CAD build for the part. Positions are in the model's coordinates, mm. A direction names the side the tool comes from. Give positions to 0.01 mm unless a question says otherwise; leave off trailing zeros. Write each loop counter-clockwise with the first axis right and the second up, starting at its lowest first coordinate (ties: lowest second). Pieces come first, ordered by that corner, then holes. Notation, with made-up numbers: M 15.25,38.5 L 37.25,38.5 A21 cw 37.25,58.5 Z; hole C 81.25,-10.75 d6. An arc over 180 degrees is marked long. One line per question, with ' | ' between items. Start each with the question number.
1. Cut at B-B, the plane x = 5. Write the cut outline in (y, z).
2. Cut at A-A, the plane z = -37.95. Write the cut outline in (x, y).
3. Cut at D-D, the plane z = -15. Write the cut outline in (x, y).
4. Pull direction Z, two halves, no side cores. Call faces 5 (the face through (6, 0, 22.75)), 6 (the face through (17, 21, -25.25)), 7 (the face through (6, 19.55, -16)): released by +Z, released by -Z, zero draft, split by the parting line, or undercut.
5. Which spindle directions (+Z, -Z, +X, -X, +Y, -Y) get a long thin tool onto all of the face, cutting with end or side? Do faces 1 (the face through (7.2, -18.8, -27.15)), 2 (the face through (10.47, 19, 6)), 3 (the face through (1, 15.35, -13)), 4 (the face through (14, 16.55, 11)). Say none if no direction does.
6. Wall check: L1, parallel to Z at x = 14.47, y = -18; L2, parallel to Y at x = 12.8, z = -24.7; L3, parallel to Z at x = 14.47, y = 18.5. Give the ranges that are in metal, low to high.
7. Cut at C-C, the plane y = 7. Write the cut outline in (x, z).
8. Flat gauge pins, fed straight in: pin 1 (3.5 mm diameter, centred on y = 22.85, z = -37.95, fed in from +X); pin 2 (3 mm diameter, centred on y = 15.5, z = -13.5, fed in from +X); pin 3 (8.5 mm diameter, centred on x = 14.5, y = -9, fed in from -Z); pin 4 (0.8 mm diameter, centred on x = 21.5, z = -23.5, fed in from -Y). Where does each tip first touch, or does it go through?
```python
from build123d import *

# Parameters (mm, degrees)
CROQUIS4_W              = 45.5
CROQUIS4_H              = 45.3
SALIENTE_EXTRUIR3_DEPTH = 21.47
CROQUIS5_W              = 41.141731218
CROQUIS5_H              = 30.7
CORTAR_EXTRUIR2_DEPTH   = 18.77
CROQUIS6_W              = 18.6
CROQUIS6_H              = 24.6
CORTAR_EXTRUIR3_DEPTH   = 18.77
CROQUIS7_R              = 3
CORTAR_EXTRUIR4_DEPTH   = 58.77
CROQUIS8_R              = 6.02
CORTAR_EXTRUIR5_DEPTH   = 58.77
CROQUIS9_W              = 6
CROQUIS9_H              = 16.319841708
CORTAR_EXTRUIR7_DEPTH   = 1.2
CHAFL_N1_SIZE           = 1.2
CROQUIS10_W             = 8
CROQUIS10_H             = 5
CORTAR_EXTRUIR8_DEPTH   = 71.2
CROQUIS11_W             = 6
CROQUIS11_H             = 16.418152186
CORTAR_EXTRUIR9_DEPTH   = 1.2
CHAFL_N2_SIZE           = 1.2
CORTAR_EXTRUIR12_DEPTH  = 11.2
CORTAR_EXTRUIR14_DEPTH  = 7
CROQUIS15_W             = 12.3
CROQUIS15_H             = 4.2
CORTAR_EXTRUIR15_DEPTH  = 9.47
CROQUIS16_W             = 7
CROQUIS16_H             = 5
CORTAR_EXTRUIR17_DEPTH  = 0.3
CROQUIS17_W             = 7
CROQUIS17_H             = 0.8
SALIENTE_EXTRUIR4_DEPTH = 3
CROQUIS18_W             = 21.819351721
CROQUIS18_H             = 12.3
CORTAR_EXTRUIR18_DEPTH  = 53
SALIENTE_EXTRUIR5_START = -2.7
CROQUIS19_W             = 24
CROQUIS19_H             = 41.5
SALIENTE_EXTRUIR5_DEPTH = 6.8
CROQUIS21_W             = 2.5
CROQUIS21_H             = 10.5
SALIENTE_EXTRUIR6_DEPTH = 20.5
CROQUIS22_R             = 1.95
CORTAR_EXTRUIR19_DEPTH  = 20.5
CROQUIS23_W             = 9.795322327
CROQUIS23_H             = 20.802243728
CORTAR_EXTRUIR20_DEPTH  = 20.5
CROQUIS24_R             = 1.1
CORTAR_EXTRUIR22_DEPTH  = 2.5
CROQUIS25_W             = 2.17
CROQUIS25_H             = 12.3
CORTAR_EXTRUIR23_DEPTH  = 13
CROQUIS26_R             = 3
CORTAR_EXTRUIR24_DEPTH  = 2.5
SALIENTE_EXTRUIR7_REACH = 70.642
CROQUIS31_W             = 4.4
CROQUIS31_H             = 7.8
SALIENTE_EXTRUIR8_DEPTH = 8.7
CROQUIS32_R             = 3
CORTAR_EXTRUIR25_DEPTH  = 8.7


# Some blends are built 0.0001 mm under size
with BuildPart() as part:
    # Croquis4 → Saliente-Extruir3 (new body)
    with BuildSketch(Plane(origin=(0, 0, 0), x_dir=(0, 0, -1), z_dir=(1, 0, 0))):
        Rectangle(CROQUIS4_W, CROQUIS4_H)
    extrude(amount=SALIENTE_EXTRUIR3_DEPTH)

    # Croquis5 → Cortar-Extruir2 (cut)
    with BuildSketch(Plane(origin=(21.47, 0, 0), x_dir=(0, 0, -1), z_dir=(1, 0, 0))):
        with Locations((2.520865609, 0)):
            Rectangle(CROQUIS5_W, CROQUIS5_H)
    extrude(amount=-CORTAR_EXTRUIR2_DEPTH, mode=Mode.SUBTRACT)

    # Croquis6 → Cortar-Extruir3 (cut)
    with BuildSketch(Plane(origin=(0, 22.65, 0), x_dir=(1, 0, 0), z_dir=(0, 1, 0))):
        with Locations((21.47, 22.75)):
            Rectangle(CROQUIS6_W, CROQUIS6_H)
    extrude(amount=-CORTAR_EXTRUIR3_DEPTH, mode=Mode.SUBTRACT)

    # Croquis7 → Cortar-Extruir4 (cut)
    with BuildSketch(Plane(origin=(0, 22.65, 0), x_dir=(1, 0, 0), z_dir=(0, 1, 0))):
        with Locations(Location((14.47, -17.25, 0), (0, 0, 270))):
            Circle(CROQUIS7_R)
        with Locations(Location((14.47, 4.95, 0), (0, 0, 270))):
            Circle(CROQUIS7_R)
    extrude(amount=-CORTAR_EXTRUIR4_DEPTH, mode=Mode.SUBTRACT)

    # Croquis8 → Cortar-Extruir5 (cut)
    with BuildSketch(Plane.XY.offset(22.75)):
        with Locations((12.7, 0)):
            Circle(CROQUIS8_R)
    extrude(amount=-CORTAR_EXTRUIR5_DEPTH, mode=Mode.SUBTRACT)

    # Croquis9 → Cortar-Extruir7 (cut)
    with BuildSketch(Plane.XZ.offset(-15.35)):
        with Locations((14.47, 6.060847086)):
            Rectangle(CROQUIS9_W, CROQUIS9_H)
    extrude(amount=-CORTAR_EXTRUIR7_DEPTH, mode=Mode.SUBTRACT)

    # Chaflán1
    # the kernel refuses this chamfer: 1.2 mm, written as the material it takes off along each edge
    with BuildSketch(Plane(origin=(12.317907402, 15.35, -2.099073768), x_dir=(0, -0.027495876610584495, -0.9996219169112968), z_dir=(1, 0, 0)), Plane(origin=(11.47, 15.35, -2.099073768), x_dir=(0, -0.027495876610584533, -0.9996219169112968), z_dir=(1, 0, 0))) as chafl_n1_piece_1:
        Polygon((CHAFL_N1_SIZE * 0.999621916911, CHAFL_N1_SIZE * 0.0274958766106), (-CHAFL_N1_SIZE * 0.0274958766106, CHAFL_N1_SIZE * 0.999621916911), (0, 0), align=None)
    extrude(amount=5.152092598, mode=Mode.SUBTRACT)
    with BuildSketch(Plane(origin=(17.47, 15.35, 14.22076794), x_dir=(0, -0.027495876610585984, 0.9996219169112968), z_dir=(-1, 0, 0))) as chafl_n1_piece_2_section:
        Polygon((CHAFL_N1_SIZE * 0.999621916911, CHAFL_N1_SIZE * 0.0274958766106), (-CHAFL_N1_SIZE * 0.0274958766106, CHAFL_N1_SIZE * 0.999621916911), (0, 0), align=None)
    chafl_n1_piece_2 = extrude(amount=6, mode=Mode.PRIVATE)
    chafl_n1_piece_2 = split(chafl_n1_piece_2, bisect_by=Plane(origin=(14.47, 16.55, 14.617252925), z_dir=(0, -1, 0)), keep=Keep.TOP, mode=Mode.PRIVATE)
    add(chafl_n1_piece_2, mode=Mode.SUBTRACT)

    # Croquis10 → Cortar-Extruir8 (cut)
    with BuildSketch(Plane(origin=(0, 22.65, 0), x_dir=(1, 0, 0), z_dir=(0, 1, 0))):
        with Locations((14.47, -6.15)):
            Rectangle(CROQUIS10_W, CROQUIS10_H)
    extrude(amount=-CORTAR_EXTRUIR8_DEPTH, mode=Mode.SUBTRACT)

    # Croquis11 → Cortar-Extruir9 (cut)
    with BuildSketch(Plane(origin=(0, -15.35, 0), x_dir=(1, 0, 0), z_dir=(0, 1, 0))):
        with Locations((14.47, -6.15)):
            Rectangle(CROQUIS11_W, CROQUIS11_H)
    extrude(amount=-CORTAR_EXTRUIR9_DEPTH, mode=Mode.SUBTRACT)

    # Chaflán2
    chafl_n2_edges = [part.edges().sort_by_distance(p)[0] for p in [
        (12.569201122, -15.35, -2.059076093),
        (16.370798878, -15.35, -2.059076093),
        (12.569201122, -15.35, 14.359076093),
        (16.370798878, -15.35, 14.359076093),
    ]]
    chamfer(chafl_n2_edges, length=CHAFL_N2_SIZE - 0.0001)  # a hair under: the kernel refuses the full size

    # Croquis12 → Cortar-Extruir12 (cut)
    with BuildSketch(Plane(origin=(2.7, 0, 0), x_dir=(0, 0, -1), z_dir=(1, 0, 0))):
        Polygon((8.65, 15.35), (8.65, -15.35), (11.55469898, -15.35), (11.55469898, -14.35), (18.45, -14.35), (18.45, 15.35), align=None)
    extrude(amount=-CORTAR_EXTRUIR12_DEPTH, mode=Mode.SUBTRACT)

    # Croquis14 → Cortar-Extruir14 (cut)
    with BuildSketch(Plane(origin=(2.7, 0, 0), x_dir=(0, 0, -1), z_dir=(1, 0, 0))):
        Polygon((10.15, 15.35), (5.15, 15.35), (10.15, 20.35), align=None)
    extrude(amount=CORTAR_EXTRUIR14_DEPTH, mode=Mode.SUBTRACT)

    # Croquis15 → Cortar-Extruir15 (cut)
    with BuildSketch(Plane(origin=(12.17, 0, 0), x_dir=(0, 0, -1), z_dir=(1, 0, 0))):
        with Locations((16.6, 17.45)):
            Rectangle(CROQUIS15_W, CROQUIS15_H)
    extrude(amount=-CORTAR_EXTRUIR15_DEPTH, mode=Mode.SUBTRACT)

    # Croquis16 → Cortar-Extruir17 (cut)
    with BuildSketch(Plane.XY.offset(-10.15)):
        with Locations((6.2, 17.85)):
            Rectangle(CROQUIS16_W, CROQUIS16_H)
    extrude(amount=-CORTAR_EXTRUIR17_DEPTH, mode=Mode.SUBTRACT)

    # Croquis17 → Saliente-Extruir4 (add)
    with BuildSketch(Plane(origin=(0, 0, -10.45), x_dir=(-1, 0, 0), z_dir=(0, 0, -1))):
        with Locations((-6.2, 19.95)):
            Rectangle(CROQUIS17_W, CROQUIS17_H)
    extrude(amount=-SALIENTE_EXTRUIR4_DEPTH)

    # Croquis18 → Cortar-Extruir18 (cut)
    with BuildSketch(Plane.XZ.offset(-19.55)):
        with Locations((13.609675861, -16.6)):
            Rectangle(CROQUIS18_W, CROQUIS18_H)
    extrude(amount=CORTAR_EXTRUIR18_DEPTH, mode=Mode.SUBTRACT)

    # Croquis19 → Saliente-Extruir5 (add)
    with BuildSketch(Plane(origin=(2.7, 0, 0), x_dir=(0, 0, -1), z_dir=(1, 0, 0)).offset(SALIENTE_EXTRUIR5_START)):
        with Locations((34.75, 5.9)):
            Rectangle(CROQUIS19_W, CROQUIS19_H)
    extrude(amount=SALIENTE_EXTRUIR5_DEPTH)

    # Croquis21 → Saliente-Extruir6 (add)
    with BuildSketch(Plane(origin=(6.8, 0, 0), x_dir=(0, 0, -1), z_dir=(1, 0, 0))):
        with Locations((24, 21.4)):
            Rectangle(CROQUIS21_W, CROQUIS21_H)
        with Locations((24, -9.6)):
            Rectangle(CROQUIS21_W, CROQUIS21_H)
    extrude(amount=SALIENTE_EXTRUIR6_DEPTH)

    # Croquis22 → Cortar-Extruir19 (cut)
    with BuildSketch(Plane(origin=(6.8, 0, 0), x_dir=(0, 0, -1), z_dir=(1, 0, 0))):
        with Locations((37.95, 22.85)):
            Circle(CROQUIS22_R)
        with Locations((37.95, -11.05)):
            Circle(CROQUIS22_R)
    extrude(amount=-CORTAR_EXTRUIR19_DEPTH, mode=Mode.SUBTRACT)

    # Croquis23 → Cortar-Extruir20 (cut)
    with BuildSketch(Plane(origin=(0, 0, -10.45), x_dir=(-1, 0, 0), z_dir=(0, 0, -1))):
        with Locations((-26.367661164, -11.870604275)):
            Rectangle(CROQUIS23_W, CROQUIS23_H)
    extrude(amount=CORTAR_EXTRUIR20_DEPTH, mode=Mode.SUBTRACT)

    # Croquis24 → Cortar-Extruir22 (cut)
    with BuildSketch(Plane(origin=(0, 0, -25.25), x_dir=(-1, 0, 0), z_dir=(0, 0, -1))):
        with Locations((-12.8, -9.25)):
            Circle(CROQUIS24_R)
        with Locations((-12.8, 19.15)):
            Circle(CROQUIS24_R)
    extrude(amount=-CORTAR_EXTRUIR22_DEPTH, mode=Mode.SUBTRACT)

    # Croquis25 → Cortar-Extruir23 (cut)
    with BuildSketch(Plane.XZ.offset(-19.55)):
        with Locations((11.085, -16.6)):
            Rectangle(CROQUIS25_W, CROQUIS25_H)
    extrude(amount=-CORTAR_EXTRUIR23_DEPTH, mode=Mode.SUBTRACT)

    # Croquis26 → Cortar-Extruir24 (cut)
    with BuildSketch(Plane(origin=(0, 0, -25.25), x_dir=(-1, 0, 0), z_dir=(0, 0, -1))):
        with Locations(Location((-22.05, 21.4, 0), (0, 0, 90))):
            Circle(CROQUIS26_R)
    extrude(amount=-CORTAR_EXTRUIR24_DEPTH, mode=Mode.SUBTRACT)

    # Saliente-Extruir7: up to this face of the body (flat: up to its plane)
    saliente_extruir7_end = Plane(part.part.faces().sort_by_distance((9.699863726, -22.65, 4.986693104))[0])
    # Croquis30 → Saliente-Extruir7 (add, up to the picked face)
    with BuildSketch(Plane.XZ.offset(-19.55), mode=Mode.PRIVATE) as saliente_extruir7_sk1:
        Polygon((2.7, -18.45), (6.8, -22.75), (2.7, -22.75), align=None)
    saliente_extruir7_tool1 = split(extrude(saliente_extruir7_sk1.sketch, amount=SALIENTE_EXTRUIR7_REACH, mode=Mode.PRIVATE), bisect_by=saliente_extruir7_end, keep=Keep.BOTH, mode=Mode.PRIVATE)
    add(saliente_extruir7_tool1.solids().sort_by(Axis((4.066667, 19.55, -21.316667), (0, -1, 0)))[0])

    # Croquis31 → Saliente-Extruir8 (add)
    with BuildSketch(Plane.ZY):
        with Locations((-24.95, -18.75)):
            Rectangle(CROQUIS31_W, CROQUIS31_H)
    extrude(amount=-SALIENTE_EXTRUIR8_DEPTH)

    # Croquis32 → Cortar-Extruir25 (cut)
    with BuildSketch(Plane(origin=(0, 0, -27.15), x_dir=(-1, 0, 0), z_dir=(0, 0, -1))):
        with Locations((-4, -18.65)):
            Circle(CROQUIS32_R)
    extrude(amount=-CORTAR_EXTRUIR25_DEPTH, mode=Mode.SUBTRACT)


solid = part.part
```
Here are the results:
1) outline: M -22.65,-27.15 L -21.48,-27.15 L -21.48,-20.86 L -22.65,-20.86 Z; M -22.65,-10.45 L -15.35,-10.45 L -15.35,18.05 L 15.35,18.05 L 15.35,-5.15 L 19.55,-9.35 L 19.55,-20.86 L -15.82,-20.86 L -15.82,-27.15 L -14.85,-27.15 L -14.85,-46.75 L 26.65,-46.75 L 26.65,-22.75 L 22.65,-22.75 L 22.65,22.75 L -22.65,22.75 Z; hole C -11.05,-37.95 d3.9; hole C 22.85,-37.95 d3.9
2) outline: M 0,-14.85 L 6.8,-14.85 L 6.8,-13 L 0,-13 Z; M 0,-9.1 L 6.8,-9.1 L 6.8,20.9 L 0,20.9 Z; M 0,24.8 L 6.8,24.8 L 6.8,26.65 L 0,26.65 Z
3) outline: M 0,-22.65 L 2.7,-22.65 L 2.7,-14.35 L 0,-14.35 Z; M 0,15.35 L 2.7,15.35 L 2.7,19.55 L 10,19.55 L 10,22.65 L 0,22.65 Z
4) face 5: released by +Z | face 6: released by -Z | face 7: undercut
5) face 1: -Z, +X, -X, -Y | face 2: +Y, -Y | face 3: +X, -X | face 4: none
6) L1: -10.45 to -7.95, -1.95 to 3.65, 8.65 to 14.25, 20.25 to 22.75 | L2: -14.85 to -10.35, -8.15 to -4.35, 16.15 to 18.05, 20.25 to 26.65 | L3: -25.25 to -22.75, -10.45 to -7.95, -1.95 to 3.65, 8.65 to 14.25, 20.25 to 22.75
7) outline: M 0,-46.75 L 6.8,-46.75 L 6.8,-22.75 L 2.7,-18.45 L 0,-18.45 Z; M 0,-8.65 L 2.7,-8.65 L 2.7,18.05 L 11.58,18.05 A3 cw 17.36,18.05 L 21.47,18.05 L 21.47,22.75 L 0,22.75 Z
8) pin 1: through | pin 2: x = 2.7 | pin 3: z = -25.25 | pin 4: y = -14.85
